from build123d import *

# Parameters (mm, degrees)
F0_W        = 114.2217256129
F0_H        = 42.490478605
F1_DEPTH    = 12.7
F2_W        = 86.1872471869
F2_H        = 15.8843388781
F3_DEPTH    = 2.54
F4_R        = 5.08
F5_SIZE     = 5.08
F6_T1_DEPTH = 39.0415311919
F7_R        = 5.08


# Not quite as in the source:
# - a fillet or chamfer that OpenCascade refuses, or shapes differently, is made with other operations: its cross-section is extruded or revolved along the edge and cut away or added


with BuildPart() as f1:
    # F0 (on Right) → F1 (new body)
    with BuildSketch(Plane.YZ):
        with Locations((10.7826646417, 2.6869159192)):
            Rectangle(F0_W, F0_H)
    extrude(amount=F1_DEPTH)

    # F2 (on face) → F3 (join)
    with BuildSketch(Plane.YZ.offset(12.7)):
        with Locations((11.4720221609, 2.5003128685)):
            Rectangle(F2_W, F2_H)
    extrude(amount=F3_DEPTH)

    # F4
    f4_edges = [f1.edges().sort_by_distance(p)[0] for p in [
        (13.97, -31.621601, 10.442482),
        (13.97, -31.621601, -5.441857),
        (13.97, 54.565646, 10.442482),
        (13.97, 54.565646, -5.441857),
    ]]
    fillet(f4_edges, radius=F4_R)

    # F5
    f5_edges = [f1.edges().sort_by_distance(p)[0] for p in [
        (6.35, 67.893527, 23.932155),
        (6.35, 67.893527, -18.558323),
        (6.35, -46.328198, -18.558323),
        (6.35, -46.328198, 23.932155),
    ]]
    chamfer(f5_edges, length=F5_SIZE)

    # F6: chamfer of 5.08 on 8 edges, made by hand

    # F6_s2 → F6_t1 (cut)
    with BuildSketch(Plane.YZ.offset(-13.170765596)):
        Polygon((-42.7360957163, 22.4442576701), (-46.3281981647, 13.7721552217), (-46.3281981647, 18.8521552217), align=None)
        Polygon((-36.1681981647, 23.9321552217), (-44.8403006131, 20.3400527733), (-41.2481981647, 23.9321552217), align=None)
        Polygon((57.7335274482, 23.9321552217), (66.4056298966, 20.3400527733), (62.8135274482, 23.9321552217), align=None)
        Polygon((64.3014249997, 22.4442576701), (67.8935274482, 13.7721552217), (67.8935274482, 18.8521552217), align=None)
        Polygon((67.8935274482, -8.3983233833), (64.3014249997, -17.0704258318), (67.8935274482, -13.4783233833), align=None)
        Polygon((66.4056298966, -14.9662209349), (57.7335274482, -18.5583233833), (62.8135274482, -18.5583233833), align=None)
        Polygon((-46.3281981647, -8.3983233833), (-42.7360957163, -17.0704258318), (-46.3281981647, -13.4783233833), align=None)
        Polygon((-44.8403006131, -14.9662209349), (-36.1681981647, -18.5583233833), (-41.2481981647, -18.5583233833), align=None)
    extrude(amount=F6_T1_DEPTH, mode=Mode.SUBTRACT)

    # F7
    f7_edges = [f1.edges().sort_by_distance(p)[0] for p in [
        (6.35, -43.352403, -15.582528),
        (6.35, -36.168198, -18.558323),
        (6.35, -46.328198, -8.398323),
        (6.35, -43.352403, 20.95636),
        (6.35, -46.328198, 13.772155),
        (6.35, -36.168198, 23.932155),
        (6.35, 57.733527, 23.932155),
        (6.35, 64.917732, 20.95636),
        (6.35, 67.893527, 13.772155),
        (6.35, 67.893527, -8.398323),
        (6.35, 64.917732, -15.582528),
        (6.35, 57.733527, -18.558323),
    ]]
    fillet(f7_edges, radius=F7_R)


solid = f1.part
Build history of the part. All positions in model axes, mm. A direction names the side the tool comes from. Coordinates: 2 decimals unless noted, no trailing zeros. Write each loop counter-clockwise with the first axis right and the second up, starting at its lowest first coordinate (ties: lowest second). Pieces come first, ordered by that corner, then holes. Notation, with made-up numbers: (-15, 21) -> (8, 21) arc R22 cw to (8, 38) -> close; hole circle Ø8 at (14.5, -6). An arc over 180 degrees is marked (long way). Use CSV: the item, a comma, the result in double quotes. Start each with the question number.
Q1. 3-axis set-ups, long thin cutter, end or side, ignore diameter. For faces 1 (the cylindrical face through (13.99, 53.12, 8.91)), 2 (the cylindrical face through (13.988, -30.094, 8.994)), 3 (the flat face through (14, 11, 10.442)): which of +Z, -Z, +X, -X, +Y, -Y reach the whole face in a straight line?
Q2. Cut at B-B, the plane y = -3.5. List the corners of the cut face in (x, z), then the cut area to 3 significant figures.
Q3. Cut at C-C, the plane z = 3. List the corners of the cut face in (x, y), then the cut area to 3 significant figures.
Q4. Drill centre lines: probe 1 along X at (y, z) = (14, -8); probe 2 along Y at (x, z) = (10.75, 14); probe 3 along Y at (x, z) = (10, 16.5). Where is each one in solid material? Low to high.
Q5. Flat gauge pins, fed straight in: pin 1 Ø4 at (x, z) = (8, 15) entering from -Y; pin 2 Ø3 at (x, z) = (14.5, 2) entering from +Y; pin 3 Ø5 at (x, y) = (13, 1.5) entering from +Z; pin 4 Ø1 at (x, z) = (11.5, 18.5) entering from +Y. Where does each tip first touch, or does it go through?
Q6. Cut at A-A, the plane x = 9.75. List the corners of the cut face in (y, z), then the cut area to 3 significant figures.
Checked values:
1,face 1,"+Z, +X, +Y"
1,face 2,"+Z, +X, -Y"
1,face 3,"+Z, +X, +Y, -Y"
2,outline,"(0, -18.56) -> (12.7, -18.56) -> (12.7, -5.44) -> (15.24, -5.44) -> (15.24, 10.44) -> (12.7, 10.44) -> (12.7, 23.93) -> (0, 23.93) -> close"
2,area,"580 mm²"
3,outline,"(0, -46.33) -> (12.7, -46.33) -> (12.7, -31.62) -> (15.24, -31.62) -> (15.24, 54.57) -> (12.7, 54.57) -> (12.7, 67.89) -> (0, 67.89) -> close"
3,area,"1,670 mm²"
4,probe 1,"x = 0 to 12.7"
4,probe 2,"y = -46.17 to 67.74"
4,probe 3,"y = -45.2 to 66.76"
5,pin 1,"stops at y = -46.32"
5,pin 2,"stops at y = 54.57"
5,pin 3,"stops at z = 23.93"
5,pin 4,"stops at y = 66.14"
6,outline,"(-46.33, -7.39) arc R5.08 ccw to (-45.94, -9.33) -> (-44.16, -13.64) arc R5.08 ccw to (-41.41, -16.39) -> (-37.1, -18.17) arc R5.08 ccw to (-35.16, -18.56) -> (56.72, -18.56) arc R5.08 ccw to (58.67, -18.17) -> (62.97, -16.39) arc R5.08 ccw to (65.72, -13.64) -> (67.51, -9.33) arc R5.08 ccw to (67.89, -7.39) -> (67.89, 12.76) arc R5.08 ccw to (67.51, 14.71) -> (65.72, 19.01) arc R5.08 ccw to (62.97, 21.76) -> (58.67, 23.55) arc R5.08 ccw to (56.72, 23.93) -> (-35.16, 23.93) arc R5.08 ccw to (-37.1, 23.55) -> (-41.41, 21.76) arc R5.08 ccw to (-44.16, 19.01) -> (-45.94, 14.71) arc R5.08 ccw to (-46.33, 12.76) -> close"
6,area,"4,730 mm²"
